from build123d import *

# Parameters (mm, degrees)
SZKIC1_R                    = 64
DODANIE_WYCI_GNI_CIE1_DEPTH = 20
SZKIC3_W                    = 1.6
SZKIC3_H                    = 3.5


with BuildPart() as part:
    # Szkic1 → Dodanie-wyciągnięcie1 (new body)
    with BuildSketch(Plane(origin=(0, 0, 0), x_dir=(1, 0, 0), z_dir=(0, 1, 0))):
        with Locations(Location((0, 0, 0), (0, 0, 270))):
            Circle(SZKIC1_R)
    extrude(amount=DODANIE_WYCI_GNI_CIE1_DEPTH)

    # Szkic3 → Wycięcie-obrót1 (revolve, cut)
    with BuildSketch(Plane(origin=(0, 0, 0), x_dir=(0, 0, -1), z_dir=(1, 0, 0)), mode=Mode.PRIVATE) as wyci_cie_obr_t1_sk:
        with Locations((-63.2, 15)):
            Rectangle(SZKIC3_W, SZKIC3_H)
        with Locations((-63.2, 5)):
            Rectangle(SZKIC3_W, SZKIC3_H)
    revolve(wyci_cie_obr_t1_sk.sketch.rotate(Axis((0, 0, 0), (0, 1, 0)), 180), axis=Axis((0, 0, 0), (0, 1, 0)), mode=Mode.SUBTRACT)


solid = part.part
Here's how the part is built. I have some questions about the finished solid (model axes, mm). A direction names the side the tool comes from. Round coordinates to 2 decimals unless told otherwise and drop trailing zeros. Order: outer loops, then holes, each group sorted by start corner. A loop starts at its lowest first (then second) coordinate and runs counter-clockwise, first axis right, second up. Notation, with made-up numbers: M 67.5,56 L 91.5,56 A14 cw 91.5,83 Z; hole C 54.5,-1 d5. An arc over 180 degrees is marked long. Return JSON: item names as keys, results as strings. Group by question number.
1. If we mould it in two halves opening along Y, with no side actions, what happens to faces 3 (the face through (-62.48, 9.95, -13.87)), 4 (the face through (1, 0, -1)), 5 (the face through (61, 3.25, -14))? For each: pulls with the +Y half, pulls with the -Y half, needs draft (parallel to the pull), parting line crosses it, or undercut.
2. On a 3-axis mill with a long thin cutter (end or side, diameter ignored), from which of +Z, -Z, +X, -X, +Y, -Y can I reach the whole of each face in a straight line? I mean faces 1 (the face through (-62.48, 1.6, -13.87)), 2 (the face through (-42.173, 5.024, 45.991)). Say none if no direction works.
3. If we section it at B-B on x = 35: List the corners of the cut face in (y, z) for me.
4. If we section it at C-C on y = 11: List the corners of the cut face in (x, z) for me, then the cut area to 3 significant figures.
5. Please list where these lines run through material, in increasing order: probe 1 along Z at (x, y) = (58.5, 10.25); probe 2 along X at (y, z) = (18.25, 38.5); probe 3 along Z at (x, y) = (-43.5, 12.5).
6. If we section it at A-A on z = 16: List the corners of the cut face in (x, y) for me, then the cut area to 3 significant figures.
7. I'm going to push flat-ended pins straight in: pin 1 Ø10 at (y, z) = (9, 21.5) entering from -X; pin 2 Ø1.5 at (y, z) = (7.5, -36) entering from -X; pin 3 Ø12 at (x, y) = (-31.5, 3) entering from +Z. Where does each tip first touch, or does it pass through?
Reply:
{
 "1": {"face 3": "needs draft", "face 4": "pulls with the -Y half", "face 5": "undercut"},
 "2": {"face 1": "+Y, -Y", "face 2": "none"},
 "3": {"outline": "M 0,-53.58 L 3.25,-53.58 L 3.25,-51.66 L 6.75,-51.66 L 6.75,-53.58 L 13.25,-53.58 L 13.25,-51.66 L 16.75,-51.66 L 16.75,-53.58 L 20,-53.58 L 20,53.58 L 16.75,53.58 L 16.75,51.66 L 13.25,51.66 L 13.25,53.58 L 6.75,53.58 L 6.75,51.66 L 3.25,51.66 L 3.25,53.58 L 0,53.58 Z"},
 "4": {"outline": "C 0,0 d128", "area": "12,900 mm^2"},
 "5": {"probe 1": "-25.96 to 25.96", "probe 2": "-51.12 to 51.12", "probe 3": "-46.94 to 46.94"},
 "6": {"outline": "M -61.97,0 L 61.97,0 L 61.97,3.25 L 60.31,3.25 L 60.31,6.75 L 61.97,6.75 L 61.97,13.25 L 60.31,13.25 L 60.31,16.75 L 61.97,16.75 L 61.97,20 L -61.97,20 L -61.97,16.75 L -60.31,16.75 L -60.31,13.25 L -61.97,13.25 L -61.97,6.75 L -60.31,6.75 L -60.31,3.25 L -61.97,3.25 Z", "area": "2,460 mm^2"},
 "7": {"pin 1": "x = -61.84", "pin 2": "x = -53.42", "pin 3": "z = 58.7"}
}
